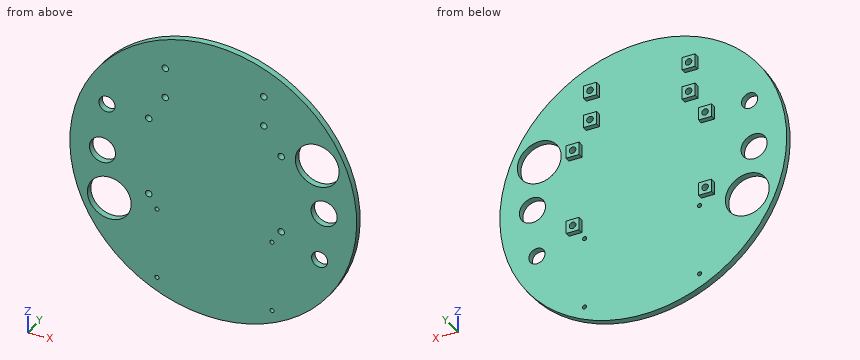
```python
from build123d import *

# Parameters (mm, degrees)
SKETCH1_R           = 69.85
SKETCH1_R_2         = 3.937
SKETCH1_R_3         = 6.35
SKETCH1_R_4         = 10.668
BOSS_EXTRUDE1_DEPTH = 3.175
SKETCH5_R           = 1.00000054
CUT_EXTRUDE1_DEPTH  = 25.4
SKETCH2_R           = 1.600000102
SKETCH2_R_2         = 1.6
CUT_EXTRUDE2_DEPTH  = 25.4
BOSS_EXTRUDE2_START = 2.54
SKETCH2_9_W         = 6.35
SKETCH2_9_H         = 6.35
SKETCH2_9_R         = 1.6
SKETCH2_9_R_2       = 1.600000102
BOSS_EXTRUDE2_DEPTH = 2.54


with BuildPart() as part:
    # Sketch1 → Boss-Extrude1 (new body)
    with BuildSketch(Plane(origin=(0, 0, 0), x_dir=(1, 0, 0), z_dir=(0, 1, 0))):
        with Locations(Location((0, 0, 0), (0, 0, 270))):
            Circle(SKETCH1_R)
        with Locations(Location((-51.795490029, -24.152633658, 0), (0, 0, 270))):
            Circle(SKETCH1_R_2, mode=Mode.SUBTRACT)
        with Locations(Location((-53.975, 0, 0), (0, 0, 270))):
            Circle(SKETCH1_R_3, mode=Mode.SUBTRACT)
        with Locations(Location((-50.64447914, 23.615908466, 0), (0, 0, 270))):
            Circle(SKETCH1_R_4, mode=Mode.SUBTRACT)
        with Locations(Location((51.795490029, 24.152633658, 0), (0, 0, 270))):
            Circle(SKETCH1_R_2, mode=Mode.SUBTRACT)
        with Locations(Location((53.975, 0, 0), (0, 0, 270))):
            Circle(SKETCH1_R_3, mode=Mode.SUBTRACT)
        with Locations(Location((50.64447914, -23.615908466, 0), (0, 0, 270))):
            Circle(SKETCH1_R_4, mode=Mode.SUBTRACT)
    extrude(amount=BOSS_EXTRUDE1_DEPTH)

    # Sketch5 → Cut-Extrude1 (cut)
    with BuildSketch(Plane(origin=(0, 3.175, 0), x_dir=(1, 0, 0), z_dir=(0, 1, 0))):
        with Locations(Location((-27.422738659, 57.298926561, 0), (0, 0, 270))):
            Circle(SKETCH5_R)
        with Locations(Location((28.577261341, 57.298926561, 0), (0, 0, 270))):
            Circle(SKETCH5_R)
        with Locations(Location((28.577261341, 22.298926561, 0), (0, 0, 270))):
            Circle(SKETCH5_R)
        with Locations(Location((-27.422738659, 22.298926561, 0), (0, 0, 270))):
            Circle(SKETCH5_R)
    extrude(amount=-CUT_EXTRUDE1_DEPTH, mode=Mode.SUBTRACT)

    # Sketch2 → Cut-Extrude2 (cut)
    with BuildSketch(Plane(origin=(0, 3.175, 0), x_dir=(1, 0, 0), z_dir=(0, 1, 0))):
        with Locations(Location((-23.404626028, -36.160958579, 0), (0, 0, 270))):
            Circle(SKETCH2_R)
        with Locations(Location((24.595373972, -36.160958579, 0), (0, 0, 270))):
            Circle(SKETCH2_R)
        with Locations(Location((-23.404626028, -51.160958579, 0), (0, 0, 270))):
            Circle(SKETCH2_R)
        with Locations(Location((24.595373972, -51.160958579, 0), (0, 0, 270))):
            Circle(SKETCH2_R)
        with Locations(Location((-31.436025901, 15.570800323, 0), (0, 0, 270))):
            Circle(SKETCH2_R_2)
        with Locations(Location((33.083974099, 15.570800323, 0), (0, 0, 270))):
            Circle(SKETCH2_R)
        with Locations(Location((-31.436025901, -23.039199677, 0), (0, 0, 270))):
            Circle(SKETCH2_R)
        with Locations(Location((33.083974099, -23.039199677, 0), (0, 0, 270))):
            Circle(SKETCH2_R)
    extrude(amount=-CUT_EXTRUDE2_DEPTH, mode=Mode.SUBTRACT)

    # Sketch2_9 → Boss-Extrude2 (add)
    # profile 1 of 8: a face of its own
    with BuildSketch(Plane(origin=(0, 3.175, 0), x_dir=(1, 0, 0), z_dir=(0, 1, 0)).offset(BOSS_EXTRUDE2_START)):
        with Locations((-31.436025901, 15.570800323)):
            Rectangle(SKETCH2_9_W, SKETCH2_9_H)
        with Locations(Location((-31.436025901, 15.570800323, 0), (0, 0, 270))):
            Circle(SKETCH2_9_R, mode=Mode.SUBTRACT)
    # profile 2 of 8: a face of its own
    with BuildSketch(Plane(origin=(0, 3.175, 0), x_dir=(1, 0, 0), z_dir=(0, 1, 0)).offset(BOSS_EXTRUDE2_START)):
        with Locations((-23.404626028, -36.160958579)):
            Rectangle(SKETCH2_9_W, SKETCH2_9_H)
        with Locations(Location((-23.404626028, -36.160958579, 0), (0, 0, 270))):
            Circle(SKETCH2_9_R_2, mode=Mode.SUBTRACT)
    # profile 3 of 8: a face of its own
    with BuildSketch(Plane(origin=(0, 3.175, 0), x_dir=(1, 0, 0), z_dir=(0, 1, 0)).offset(BOSS_EXTRUDE2_START)):
        with Locations((24.595373972, -36.160958579)):
            Rectangle(SKETCH2_9_W, SKETCH2_9_H)
        with Locations(Location((24.595373972, -36.160958579, 0), (0, 0, 270))):
            Circle(SKETCH2_9_R_2, mode=Mode.SUBTRACT)
    # profile 4 of 8: a face of its own
    with BuildSketch(Plane(origin=(0, 3.175, 0), x_dir=(1, 0, 0), z_dir=(0, 1, 0)).offset(BOSS_EXTRUDE2_START)):
        with Locations((-23.404626028, -51.160958579)):
            Rectangle(SKETCH2_9_W, SKETCH2_9_H)
        with Locations(Location((-23.404626028, -51.160958579, 0), (0, 0, 270))):
            Circle(SKETCH2_9_R_2, mode=Mode.SUBTRACT)
    # profile 5 of 8: a face of its own
    with BuildSketch(Plane(origin=(0, 3.175, 0), x_dir=(1, 0, 0), z_dir=(0, 1, 0)).offset(BOSS_EXTRUDE2_START)):
        with Locations((24.595373972, -51.160958579)):
            Rectangle(SKETCH2_9_W, SKETCH2_9_H)
        with Locations(Location((24.595373972, -51.160958579, 0), (0, 0, 270))):
            Circle(SKETCH2_9_R_2, mode=Mode.SUBTRACT)
    # profile 6 of 8: a face of its own
    with BuildSketch(Plane(origin=(0, 3.175, 0), x_dir=(1, 0, 0), z_dir=(0, 1, 0)).offset(BOSS_EXTRUDE2_START)):
        with Locations((-31.436025901, -23.039199677)):
            Rectangle(SKETCH2_9_W, SKETCH2_9_H)
        with Locations(Location((-31.436025901, -23.039199677, 0), (0, 0, 270))):
            Circle(SKETCH2_9_R_2, mode=Mode.SUBTRACT)
    # profile 7 of 8: a face of its own
    with BuildSketch(Plane(origin=(0, 3.175, 0), x_dir=(1, 0, 0), z_dir=(0, 1, 0)).offset(BOSS_EXTRUDE2_START)):
        with Locations((33.083974099, -23.039199677)):
            Rectangle(SKETCH2_9_W, SKETCH2_9_H)
        with Locations(Location((33.083974099, -23.039199677, 0), (0, 0, 270))):
            Circle(SKETCH2_9_R_2, mode=Mode.SUBTRACT)
    # profile 8 of 8: a face of its own
    with BuildSketch(Plane(origin=(0, 3.175, 0), x_dir=(1, 0, 0), z_dir=(0, 1, 0)).offset(BOSS_EXTRUDE2_START)):
        with Locations((33.083974099, 15.570800323)):
            Rectangle(SKETCH2_9_W, SKETCH2_9_H)
        with Locations(Location((33.083974099, 15.570800323, 0), (0, 0, 270))):
            Circle(SKETCH2_9_R_2, mode=Mode.SUBTRACT)
    extrude(amount=-BOSS_EXTRUDE2_DEPTH)


solid = part.part
```
Could you check a few things on this model? Use its own coordinates, in mm. Coordinates: 2 decimals unless noted, no trailing zeros. Loops run counter-clockwise (first coordinate to the right, second up) from the corner with the lowest first, then second, coordinate; pieces in that order, holes last.
1) Imagine slicing it at A-A (z = 0). List the corners of the cut face in (x, y) for me (3 decimals), and give its area (3 significant figures).
Reported:
outline: (-69.85, 0) - (-60.325, 0) - (-60.325, 3.175) - (-69.85, 3.175) - close; (-47.625, 0) - (47.625, 0) - (47.625, 3.175) - (-47.625, 3.175) - close; (60.325, 0) - (69.85, 0) - (69.85, 3.175) - (60.325, 3.175) - close
area: 363 mm2
2) Imagine slicing it at D-D (x = 0). List the corners of the cut face in (y, z) for me (3 decimals), and give its area (3 significant figures).
Reported:
outline: (0, -69.85) - (3.175, -69.85) - (3.175, 69.85) - (0, 69.85) - close
area: 444 mm2
3) Please list where these lines run through material, in increasing order: line 1 along X through (y, z) = (1.35, 0) (3 decimals); line 2 along Z through (x, y) = (30.5, 4.85); line 3 along Z through (x, y) = (-59, 1.8).
Reported:
line 1: x = -69.85 to -60.325, -47.625 to 47.625, 60.325 to 69.85
line 2: z = -18.75 to -12.4, 19.86 to 26.21
line 3: z = -37.39 to -30.25, -16.98 to -3.88, 3.88 to 37.39
4) Imagine slicing it at B-B (y = 1.9). State how many separate pieces and enclosed holes the cut face has, and give its area (3 significant figures).
Reported:
separate pieces: 1
enclosed holes: 18
area: 14,200 mm2
5) Will these pins go through, and if not, where does the flat tip stop? pin 1 Ø1.3 at (y, z) = (4, 36.5) entering from -X; pin 2 Ø10 at (x, z) = (51.8, -24.15) entering from -Y; pin 3 Ø3 at (x, z) = (-31.44, -15.57) entering from +Y; pin 4 Ø1.3 at (y, z) = (4.5, 36.5) entering from +X.
Reported:
pin 1: stops at x = -26.58
pin 2: stops at y = 0
pin 3: passes through
pin 4: stops at x = 27.77
6) Imagine slicing it at C-C (x = -44.5). List the corners of the cut face in (y, z) for me (3 decimals).
Reported:
outline: (0, -53.84) - (3.175, -53.84) - (3.175, -32.337) - (0, -32.337) - close; (0, -14.895) - (3.175, -14.895) - (3.175, 53.84) - (0, 53.84) - close
